from build123d import *

# Parameters (mm, degrees)
SKETCH2_R           = 5.08
BOSS_EXTRUDE2_DEPTH = 41.91
SKETCH8_W           = 50.8
SKETCH8_H           = 177.8
BOSS_EXTRUDE3_DEPTH = 10.16
SKETCH11_W          = 41.599124914
SKETCH11_H          = 41.599124914
SKETCH11_R          = 12.5
BOSS_EXTRUDE6_DEPTH = 2.54
CUT_EXTRUDE1_DEPTH  = 25
SKETCH14_R          = 1.5
SKETCH14_R_2        = 3.81
CUT_EXTRUDE5_DEPTH  = 30.94
SKETCH18_R          = 12.5
CUT_EXTRUDE6_DEPTH  = 3
SKETCH19_W          = 42.604525883
SKETCH19_H          = 46.988260705
CUT_EXTRUDE7_DEPTH  = 85.804


with BuildPart() as part:
    # Sketch2 → Boss-Extrude2 (new body)
    with BuildSketch(Plane(origin=(0, 0, 0), x_dir=(-1, 0, 0), z_dir=(0, 1, 0))):
        with Locations(Location((0, 0, 0), (0, 0, 90))):
            Circle(SKETCH2_R)
    extrude(amount=BOSS_EXTRUDE2_DEPTH)

    # Sketch8 → Boss-Extrude3 (add)
    with BuildSketch(Plane(origin=(0, 41.91, 0), x_dir=(1, 0, 0), z_dir=(0, 1, 0))):
        with Locations((0, -65.27767655)):
            Rectangle(SKETCH8_W, SKETCH8_H)
    extrude(amount=BOSS_EXTRUDE3_DEPTH)

    # Sketch11 → Boss-Extrude6 (add)
    with BuildSketch(Plane(origin=(0, 52.07, 0), x_dir=(1, 0, 0), z_dir=(0, 1, 0))):
        Rectangle(SKETCH11_W, SKETCH11_H)
        with Locations(Location((0, 0, 0), (0, 0, 270))):
            Circle(SKETCH11_R, mode=Mode.SUBTRACT)
    extrude(amount=BOSS_EXTRUDE6_DEPTH)

    # Sketch12 → Cut-Extrude1 (cut)
    with BuildSketch(Plane(origin=(0, 52.07, 0), x_dir=(1, 0, 0), z_dir=(0, 1, 0))):
        with BuildLine():
            Line((2.628413525, 0.246153039), (0.602559077, 2.570227915))
            ThreePointArc((0.602559077, 2.570227915), (-2.068798379, -1.639884826), (2.639914577, 0))
            ThreePointArc((2.639914577, 0), (2.637037747, 0.123210788), (2.628413525, 0.246153039))
        make_face()
    extrude(amount=-CUT_EXTRUDE1_DEPTH, mode=Mode.SUBTRACT)

    # Sketch14 → Cut-Extrude5 (cut)
    with BuildSketch(Plane.XZ.offset(-41.91)):
        with Locations(Location((15.5, 144.27767655, 0), (0, 0, 270))):
            Circle(SKETCH14_R)
        with Locations(Location((0, 128.77767655, 0), (0, 0, 270))):
            Circle(SKETCH14_R_2)
        with Locations(Location((-15.5, 113.27767655, 0), (0, 0, 270))):
            Circle(SKETCH14_R)
        with Locations(Location((15.5, 113.27767655, 0), (0, 0, 270))):
            Circle(SKETCH14_R)
        with Locations(Location((-15.5, 144.27767655, 0), (0, 0, 270))):
            Circle(SKETCH14_R)
    extrude(amount=-CUT_EXTRUDE5_DEPTH, mode=Mode.SUBTRACT)

    # Sketch18 → Cut-Extrude6 (cut)
    with BuildSketch(Plane(origin=(0, 52.07, 0), x_dir=(1, 0, 0), z_dir=(0, 1, 0))):
        with Locations(Location((0, -128.77767655, 0), (0, 0, 270))):
            Circle(SKETCH18_R)
    extrude(amount=-CUT_EXTRUDE6_DEPTH, mode=Mode.SUBTRACT)

    # Sketch19 → Cut-Extrude7 (cut)
    with BuildSketch(Plane.ZY.offset(25.4)):
        with Locations((-1.112784187, 18.415869648)):
            Rectangle(SKETCH19_W, SKETCH19_H)
    extrude(amount=-CUT_EXTRUDE7_DEPTH, mode=Mode.SUBTRACT)


solid = part.part
Work out the finished part from the listing and answer in its coordinate system (mm). A direction names the side the tool comes from. Give positions to 0.01 mm unless a question says otherwise; leave off trailing zeros. Order: outer loops, then holes, each group sorted by start corner. A loop starts at its lowest first (then second) coordinate and runs counter-clockwise, first axis right, second up. Notation, with made-up numbers: M 87,-20.75 L 146,-20.75 A17 ccw 146,5.25 Z; hole C 4.25,28 d6. An arc over 180 degrees is marked long. Return JSON: item names as keys, results as strings.
Q1. Find section D-D, the plane z = 49. Write down the section's boundary in (x, y).
Answer below:
{"outline": "M -25.4,41.91 L 25.4,41.91 L 25.4,52.07 L -25.4,52.07 Z"}
Q2. Find section A-A, the plane x = -15.5. Write down the section's boundary in (y, z).
Answer below:
{"outline": "M 41.91,-23.62 L 52.07,-23.62 L 52.07,-20.8 L 54.61,-20.8 L 54.61,20.8 L 52.07,20.8 L 52.07,111.78 L 41.91,111.78 Z; M 41.91,114.78 L 52.07,114.78 L 52.07,142.78 L 41.91,142.78 Z; M 41.91,145.78 L 52.07,145.78 L 52.07,154.18 L 41.91,154.18 Z"}
Q3. Find section C-C, the plane z = 123. Write down the section's boundary in (x, y), and give its area (3 significant figures).
Answer below:
{"outline": "M -25.4,41.91 L 25.4,41.91 L 25.4,52.07 L 11.08,52.07 L 11.08,49.07 L -11.08,49.07 L -11.08,52.07 L -25.4,52.07 Z", "area": "450 mm^2"}
Q4. Which of the six approach directions +Z, -Z, +X, -X, +Y, -Y give full straight-line access (tool end or side, diameter ignored) to faces 1 (the face through (0.55, 50.59, 116.29)), 2 (the face through (0, 47, 154.178))?
Answer below:
{"face 1": "+Y", "face 2": "+Z, +X, -X, +Y, -Y"}
Q5. Find section B-B, the plane x = 19. Write down the section's boundary in (y, z), and give its area (3 significant figures).
Answer below:
{"outline": "M 41.91,-23.62 L 52.07,-23.62 L 52.07,-20.8 L 54.61,-20.8 L 54.61,20.8 L 52.07,20.8 L 52.07,154.18 L 41.91,154.18 Z", "area": "1,910 mm^2"}
Q6. Each of these flat-tipped pins is pushed along its axis until it touches: pin 1 (22.5 mm diameter, centred on x = 0, z = 0, fed in from -Y); pin 2 (3.5 mm diameter, centred on x = -15.5, z = 144.28, fed in from +Y); pin 3 (0.8 mm diameter, centred on y = 53, z = -3, fed in from +X); pin 4 (0.8 mm diameter, centred on y = 53.5, z = -2, fed in from -X). Where does it stop, or does it pass through?
Answer below:
{"pin 1": "stops at y = 41.91", "pin 2": "stops at y = 52.07", "pin 3": "stops at x = 20.8", "pin 4": "stops at x = -20.8"}
Q7. The mould has two halves that part along Z. Classify faces 3 (the face through (0, 47, -23.622)), 4 (the face through (3.755, 53.322, 11.923)), 5 (the face through (0, 41.91, 64)): pulls with the +Z half, pulls with the -Z half, needs draft (parallel to the pull), parting line crosses it, or undercut.
Answer below:
{"face 3": "pulls with the -Z half", "face 4": "undercut", "face 5": "needs draft"}
Q8. Find the intervals of material crossed by line 1 along X through (y, z) = (48.25, 144.5); line 2 along X through (y, z) = (53.3, 0); line 3 along Y through (x, z) = (14, 78.5), in increasing order. Write a range as [from, to].
Answer below:
{"line 1": "x = [-25.4, -16.98], [-14.02, 14.02], [16.98, 25.4]", "line 2": "x = [-20.8, -12.5], [12.5, 20.8]", "line 3": "y = [41.91, 52.07]"}
